```python
from build123d import *

# Parameters (mm, degrees)
SKETCH1_W                      = 9.525
SKETCH1_H                      = 19.05
SKETCH1_W_2                    = 3.175
BOSS_EXTRUDE1_DEPTH            = 3.175
BOSS_EXTRUDE2_START            = 3.175
SKETCH1_3_W                    = 3.175
SKETCH1_3_H                    = 19.05
BOSS_EXTRUDE2_DEPTH            = 12.7
SKETCH2_R                      = 2
CUT_EXTRUDE1_DEPTH             = 21.819867315
SKETCH4_W                      = 12.7
SKETCH4_H                      = 45.72
BOSS_EXTRUDE3_DEPTH            = 22.225
SKETCH3_R                      = 12.7
CUT_EXTRUDE2_DEPTH             = 48.21685107
F_8_0_199_DIAMETER_HOLE1_D     = 5.0546
F_8_0_199_DIAMETER_HOLE1_DEPTH = 61.468
F_8_0_199_DIAMETER_HOLE1_TIP   = 1.518555042


with BuildPart() as part:
    # Sketch1 → Boss-Extrude1 (new body)
    with BuildSketch(Plane(origin=(0, 0, 0), x_dir=(1, 0, 0), z_dir=(0, 1, 0))):
        with Locations((1.5875, 0)):
            Rectangle(SKETCH1_W, SKETCH1_H)
        with Locations((-4.7625, 0)):
            Rectangle(SKETCH1_W_2, SKETCH1_H)
    extrude(amount=BOSS_EXTRUDE1_DEPTH)

    # Sketch1<3> → Boss-Extrude2 (add)
    with BuildSketch(Plane(origin=(0, 0, 0), x_dir=(1, 0, 0), z_dir=(0, 1, 0)).offset(BOSS_EXTRUDE2_START)):
        with Locations((-4.7625, 0)):
            Rectangle(SKETCH1_3_W, SKETCH1_3_H)
    extrude(amount=BOSS_EXTRUDE2_DEPTH)

    # Sketch2 → Cut-Extrude1 (cut, through all)
    with BuildSketch(Plane(origin=(-3.175, 0, 0), x_dir=(0, 0, -1), z_dir=(1, 0, 0))):
        with Locations((0, 12.7)):
            Circle(SKETCH2_R)
    extrude(amount=-CUT_EXTRUDE1_DEPTH, mode=Mode.SUBTRACT)

    # Sketch4 → Boss-Extrude3 (add)
    with BuildSketch(Plane.XZ):
        with Locations((12.7, 10.16)):
            Rectangle(SKETCH4_W, SKETCH4_H)
    extrude(amount=-BOSS_EXTRUDE3_DEPTH)

    # Sketch3 → Cut-Extrude2 (cut, through all)
    with BuildSketch(Plane.ZY.offset(6.35)):
        with Locations((10.606601718, 23.306601718)):
            Circle(SKETCH3_R)
    extrude(amount=-CUT_EXTRUDE2_DEPTH, mode=Mode.SUBTRACT)

    # #8 (0.199) Diameter Hole1
    with Locations(Plane(origin=(0, 22.225, 0), x_dir=(1, 0, 0), z_dir=(0, 1, 0))):
        with Locations((12.7, 8.868531542), (12.7, -30.047302209)):
            Hole(F_8_0_199_DIAMETER_HOLE1_D / 2, depth=F_8_0_199_DIAMETER_HOLE1_DEPTH)
            with Locations((0, 0, -(F_8_0_199_DIAMETER_HOLE1_DEPTH + F_8_0_199_DIAMETER_HOLE1_TIP / 2))):  # 118° drill point
                Cone(0, F_8_0_199_DIAMETER_HOLE1_D / 2, F_8_0_199_DIAMETER_HOLE1_TIP, mode=Mode.SUBTRACT)


solid = part.part
```
Read the model definition and answer for the solid it produces. Units are mm, in the model's axes. A direction names the side the tool comes from. Give positions to 0.01 mm unless a question says otherwise; leave off trailing zeros. Loops run counter-clockwise (first coordinate to the right, second up) from the corner with the lowest first, then second, coordinate; pieces in that order, holes last.
Item 1: The mould has two halves that part along Y. Classify faces 1 (the cylindrical face through (15.225, 10.957, 29.936)), 2 (the cylindrical face through (-4.785, 12.295, 4.28)), 3 (the cylindrical face through (-4.74, 10.748, 0.434)), 4 (the flat face through (9, 0, 5)): released by +Y, released by -Y, zero draft, split by the parting line, or undercut.
Item 2: Each of these flat-tipped pins is pushed along its axis until it touches: pin 1 Ø8 at (x, z) = (3, 24) entering from -Y; pin 2 Ø10 at (x, y) = (-0.5, 6.5) entering from -Z (3 decimals); pin 3 Ø10.5 at (x, z) = (-0.5, 1.5) entering from +Y (3 decimals); pin 4 Ø6.5 at (y, z) = (15.5, 16.5) entering from -X. Where does it stop, or does it pass through?
Item 3: Find the intervals of material crossed by line 1 along Z through (x, y) = (12.7, 10); line 2 along X through (y, z) = (9.25, 30); line 3 along Z through (x, y) = (12.7, 15), in increasing order.
Item 4: The part is cut by section B-B (x = 12.7). Write down the section's boundary in (y, z) (3 decimals).
Item 5: For faces 5 (the flat face through (-4, 4, -9.525)), 6 (the flat face through (2, 3.175, 0)), 7 (the flat face through (-2, 3, 9.525)), 8 (the flat face through (-5, 15.875, -5)), determine the directions among +Z, -Z, +X, -X, +Y, -Y from which every point of the face is accessible in a straight line to the end or side of a thin tool.
Item 6: The part is cut by section D-D (z = -4). Write down the section's boundary in (x, y) (3 decimals), and give its area (3 significant figures).
Item 7: The part is cut by section C-C (y = 17.75). Write down the section's boundary in (x, z).
Item 8: The part is cut by section A-A (y = 11.75). Write down the section's boundary in (x, z) (3 decimals), and give its area (3 significant figures).
Taken from the geometry:
1. face 1: zero draft
1. face 2: released by +Y
1. face 3: undercut
1. face 4: released by -Y
2. pin 1: stops at y = 0
2. pin 2: stops at z = -9.525
2. pin 3: stops at y = 15.875
2. pin 4: stops at x = 6.35
3. line 1: z = -12.7 to -11.4, -6.34 to 27.52, 32.57 to 33.02
3. line 2: x = 6.35 to 10.17, 15.23 to 19.05
3. line 3: z = -12.7 to -11.4, -6.34 to 1, 20.21 to 27.52, 32.57 to 33.02
4. outline: (0, -12.7) - (22.225, -12.7) - (22.225, -11.396) - (0, -11.396) - close; (0, -6.341) - (22.225, -6.341) - (22.225, -2.047) arc R12.7 cw to (22.225, 23.26) - (22.225, 27.52) - (0, 27.52) - close; (0, 32.575) - (22.225, 32.575) - (22.225, 33.02) - (0, 33.02) - close
5. face 5: -Z, -X, +Y, -Y
5. face 6: +Z, -Z, +Y
5. face 7: +Z, -X, +Y, -Y
5. face 8: +Z, -Z, -X, +Y
6. outline: (-6.35, 0) - (19.05, 0) - (19.05, 22.225) - (6.35, 22.225) - (6.35, 3.175) - (-3.175, 3.175) - (-3.175, 15.875) - (-6.35, 15.875) - close
6. area: 363 mm2
7. outline: (6.35, -12.7) - (19.05, -12.7) - (19.05, -0.81) - (6.35, -0.81) - close; (6.35, 22.03) - (19.05, 22.03) - (19.05, 33.02) - (6.35, 33.02) - close; hole circle Ø5.05 at (12.7, -8.87); hole circle Ø5.05 at (12.7, 30.05)
8. outline: (-6.35, -9.525) - (-3.175, -9.525) - (-3.175, -1.76) - (-6.35, -1.76) - close; (-6.35, 1.76) - (-3.175, 1.76) - (-3.175, 5.34) - (-6.35, 5.34) - close; (6.35, -12.7) - (19.05, -12.7) - (19.05, 5.34) - (6.35, 5.34) - close; (6.35, 15.873) - (19.05, 15.873) - (19.05, 33.02) - (6.35, 33.02) - close; hole circle Ø5.055 at (12.7, -8.869); hole circle Ø5.055 at (12.7, 30.047)
8. area: 443 mm2
